Check sheet for the modelled part. Datum: model origin and axes. Units: mm. A direction names the side the tool comes from. Round coordinates to 2 decimals unless told otherwise and drop trailing zeros. Order: outer loops, then holes, each group sorted by start corner. A loop starts at its lowest first (then second) coordinate and runs counter-clockwise, first axis right, second up.
Autodesk Inventor part; units mm, degrees
ref_plane "YZ Plane" through (0, 0, 0) normal (1, 0, 0) x (0, 1, 0)
ref_plane "XZ Plane" through (0, 0, 0) normal (0, 1, 0) x (-1, 0, 0)
ref_plane "XY Plane" through (0, 0, 0) normal (0, 0, 1) x (1, 0, 0)
ref_plane "Arbeitsebene7" through (0, 0, 0) normal (0, 0, 1) x (1, 0, 0)
sketch "Skizze1" plane through (0, 0, 0) normal (0, 0, 1) x (1, 0, 0)
  line L0 (12, 20) -> (17, 20)
  line L1 (0, 20) -> (5, 20)
  line L2 (17, 20) -> (0, 20)
  line L3 (0, 20) -> (0, 40)
  line L4 (0, 40) -> (17, 40)
  line L5 (17, 40) -> (17, 20)
  point P0 (0, 0)
  dimension "d0" = 20
extrude "Extrusion1" add sketch "Skizze1" along normal blind 3
ref_plane "Arbeitsebene6" through (5, 20, 0) normal (0, 1, 0) x (-1, 0, 0)
sketch "Skizze2" plane through (5, 20, 0) normal (0, 1, 0) x (-1, 0, 0)
  line L0 (-12, 0) -> (-12, 400)
  line L1 (5, 3) -> (-12, 3)
  line L2 (-12, 3) -> (5, 3)
  line L3 (5, 3) -> (5, 20)
  line L4 (5, 20) -> (-12, 20)
  line L5 (-12, 20) -> (-12, 3)
  point P0 (5, 0)
  dimension "d3" = 17
extrude "Extrusion2" add sketch "Skizze2" along normal blind 3
ref_plane "Arbeitsebene5" through (0, 20, 0) normal (-1, 0, 0) x (0, 0, 1)
sketch "Skizze4" plane through (0, 20, 0) normal (-1, 0, 0) x (0, 0, 1)
  line L0 (3, 3) -> (3, 20)
  line L1 (20, 3) -> (3, 3)
  line L2 (3, 20) -> (20, 3)
  line L3 (20, 3) -> (3, 3)
  line L4 (0, 20) -> (3, 20)
  line L5 (3, 3) -> (3, 20)
  point P0 (0, -20)
extrude "Extrusion3" add sketch "Skizze4" against normal blind 3
ref_plane "Arbeitsebene4" through (17, 20, 0) normal (1, 0, 0) x (0, 0, -1)
sketch "Skizze5" plane through (17, 20, 0) normal (1, 0, 0) x (0, 0, -1)
  line L0 (-3, 3) -> (-3, 20)
  line L1 (-3, 20) -> (-3, 3)
  line L2 (-20, 3) -> (-3, 3)
  line L3 (-3, 3) -> (-20, 3)
  line L4 (-3, 20) -> (-20, 3)
  line L5 (-20, 3) -> (-3, 20)
  point P0 (0, -20)
extrude "Extrusion4" add sketch "Skizze5" against normal blind 3
hole "Bohrung3" at (8.5, 30, 3) direction (0, 0, -1) diameter 6 end through all
hole "Bohrung4" at (8.5, 23, 10) direction (0, -1, 0) diameter 6 end through all
properties part number "Corner Piece" material "Aluminum 6061-AHC"
Item 1: Sectioned sample at A-A (x = 8.5). Record the cut outline in (y, z).
Answer:
outline: (20, 0) - (27, 0) - (27, 3) - (23, 3) - (23, 7) - (20, 7) - close; (20, 13) - (23, 13) - (23, 20) - (20, 20) - close; (33, 0) - (40, 0) - (40, 3) - (33, 3) - close
Item 2: Go/stop test with flat-tipped pins: P1, Ø9.5, axis at x = 8.5, y = 30, coming from the +Z side; P2, Ø8, axis at x = 9, y = 29.5, coming from the -Z side; P3, Ø1.5, axis at x = 13.5, z = 17, coming from the +Y side. Record where each tip stops, or that it passes through.
Answer:
P1: stops at z = 3
P2: stops at z = 0
P3: stops at y = 26.56
Item 3: Sectioned sample at D-D (y = 35). Record the cut outline in (x, z), and give its area (3 significant figures).
Answer:
outline: (0, 0) - (17, 0) - (17, 8) - (14, 8) - (14, 3) - (3, 3) - (3, 8) - (0, 8) - close
area: 81.0 mm2
Item 4: Scan lines: line 1 along X through (y, z) = (21.3, 10); line 2 along X through (y, z) = (28.25, 12.25); line 3 along Y through (x, z) = (8.5, 1.05). Record each from-to range of solid material in increasing order.
Answer:
line 1: x = 0 to 5.5, 11.5 to 17
line 2: x = 0 to 3, 14 to 17
line 3: y = 20 to 27, 33 to 40
Item 5: Access from +Z, -Z, +X, -X, +Y, -Y to the whole of each face (thin tool, end or side, straight path). Record for faces 4 (the flat face through (1, 32, 11)), 5 (the flat face through (8, 34, 3)).
Answer:
face 4: +Z, +X, -X, +Y
face 5: +Z, +Y
Item 6: Sectioned sample at C-C (z = 10). Record the cut outline in (x, y), and give its area (3 significant figures).
Answer:
outline: (0, 20) - (5.5, 20) - (5.5, 23) - (3, 23) - (3, 33) - (0, 33) - close; (11.5, 20) - (17, 20) - (17, 33) - (14, 33) - (14, 23) - (11.5, 23) - close
area: 93.0 mm2
Item 7: Release check for a two-part mould opening along X. For faces 1 (the flat face through (9, 23, 14)), 2 (the flat face through (0, 28, 8)), 3 (the flat face through (6, 32, 0)) record: released by +X, released by -X, zero draft, split by the parting line, or undercut.
Answer:
face 1: undercut
face 2: released by -X
face 3: zero draft
Item 8: Sectioned sample at B-B (y = 30). Record the cut outline in (x, z), and give its area (3 significant figures).
Answer:
outline: (0, 0) - (5.5, 0) - (5.5, 3) - (3, 3) - (3, 13) - (0, 13) - close; (11.5, 0) - (17, 0) - (17, 13) - (14, 13) - (14, 3) - (11.5, 3) - close
area: 93.0 mm2
